CAD build for the part. Positions are in the model's coordinates, mm. A direction names the side the tool comes from. Round coordinates to 2 decimals unless told otherwise and drop trailing zeros. Order: outer loops, then holes, each group sorted by start corner. A loop starts at its lowest first (then second) coordinate and runs counter-clockwise, first axis right, second up. Notation, with made-up numbers: M 76,46.25 L 125,46.25 A22 cw 125,62.25 Z; hole C 87.5,-15 d4. An arc over 180 degrees is marked long. Answer as a JSON object with one key per item and string values.
```python
from build123d import *

# Parameters (mm, degrees)
SKETCH1_W                      = 74.3
SKETCH1_H                      = 60
BOSS_EXTRUDE1_DEPTH            = 1.6
SKETCH2_W                      = 1.9
SKETCH2_H                      = 15
CUT_EXTRUDE1_DEPTH             = 2.6
F_3_2_3_2_DIAMETER_HOLE1_D     = 3.2
F_3_2_3_2_DIAMETER_HOLE1_DEPTH = 60
F_3_2_3_2_DIAMETER_HOLE1_TIP   = 0.96137699
SKETCH6_W                      = 70.5
SKETCH6_H                      = 45
BOSS_EXTRUDE2_DEPTH            = 2
SKETCH7_W                      = 57.288
SKETCH7_H                      = 38.192
BOSS_EXTRUDE3_DEPTH            = 0.5


with BuildPart() as part:
    # Sketch1 → Boss-Extrude1 (new body)
    with BuildSketch(Plane.XY):
        with Locations((37.15, 30)):
            Rectangle(SKETCH1_W, SKETCH1_H)
    extrude(amount=BOSS_EXTRUDE1_DEPTH)

    # Sketch2 → Cut-Extrude1 (cut, through all)
    with BuildSketch(Plane.XY.offset(1.6)):
        with Locations((0.95, 15)):
            Rectangle(SKETCH2_W, SKETCH2_H)
    extrude(amount=-CUT_EXTRUDE1_DEPTH, mode=Mode.SUBTRACT)

    # Ø3.2 (3.2) Diameter Hole1
    with Locations(Plane.XY.offset(1.6)):
        with Locations((4, 56), (70.3, 56), (70.3, 4), (4, 4)):
            Hole(F_3_2_3_2_DIAMETER_HOLE1_D / 2, depth=F_3_2_3_2_DIAMETER_HOLE1_DEPTH)
            with Locations((0, 0, -(F_3_2_3_2_DIAMETER_HOLE1_DEPTH + F_3_2_3_2_DIAMETER_HOLE1_TIP / 2))):  # 118° drill point
                Cone(0, F_3_2_3_2_DIAMETER_HOLE1_D / 2, F_3_2_3_2_DIAMETER_HOLE1_TIP, mode=Mode.SUBTRACT)

    # Sketch6 → Boss-Extrude2 (add)
    with BuildSketch(Plane.XY.offset(1.6)):
        with Locations((37.15, 30)):
            Rectangle(SKETCH6_W, SKETCH6_H)
    extrude(amount=BOSS_EXTRUDE2_DEPTH)

    # Sketch7 → Boss-Extrude3 (add)
    with BuildSketch(Plane.XY.offset(3.6)):
        with Locations((39.936, 30)):
            Rectangle(SKETCH7_W, SKETCH7_H)
    extrude(amount=BOSS_EXTRUDE3_DEPTH)


solid = part.part
```
Item 1: Saw through at A-A on x = 70.3. List the corners of the cut face in (y, z).
Worked answers:
{"outline": "M 0,0 L 2.4,0 L 2.4,1.6 L 0,1.6 Z; M 5.6,0 L 54.4,0 L 54.4,1.6 L 52.5,1.6 L 52.5,3.6 L 7.5,3.6 L 7.5,1.6 L 5.6,1.6 Z; M 57.6,0 L 60,0 L 60,1.6 L 57.6,1.6 Z"}
Item 2: Saw through at D-D on y = 28. List the corners of the cut face in (x, z), and give its area (3 significant figures).
Worked answers:
{"outline": "M 0,0 L 74.3,0 L 74.3,1.6 L 72.4,1.6 L 72.4,3.6 L 68.58,3.6 L 68.58,4.1 L 11.29,4.1 L 11.29,3.6 L 1.9,3.6 L 1.9,1.6 L 0,1.6 Z", "area": "289 mm2"}
Item 3: Wall check: line 1 along Y through (x, z) = (70.3, 0.7); line 2 along Z through (x, y) = (49, 8.5); line 3 along Z through (x, y) = (13, 4). Give the ranges that are in metal, low to high. Write a range as [from, to].
Worked answers:
{"line 1": "y = [0, 2.4], [5.6, 54.4], [57.6, 60]", "line 2": "z = [0, 3.6]", "line 3": "z = [0, 1.6]"}
Item 4: 3-axis set-ups, long thin cutter, end or side, ignore diameter. For faces 4 (the flat face through (1, 7.5, 1)), 5 (the flat face through (37, 52.5, 3)), 6 (the flat face through (37, 7.5, 3)), 7 (the cylindrical face through (71.9, 4.07, 0.79)): which of +Z, -Z, +X, -X, +Y, -Y reach the whole face in a straight line?
Worked answers:
{"face 4": "+Z, -Z, -X", "face 5": "+Z, +X, -X, +Y", "face 6": "+Z, +X, -X, -Y", "face 7": "+Z, -Z"}
Item 5: Saw through at B-B on y = 56. List the corners of the cut face in (x, z).
Worked answers:
{"outline": "M 0,0 L 2.4,0 L 2.4,1.6 L 0,1.6 Z; M 5.6,0 L 68.7,0 L 68.7,1.6 L 5.6,1.6 Z; M 71.9,0 L 74.3,0 L 74.3,1.6 L 71.9,1.6 Z"}
Item 6: Two-plate mould, pull along X, no slides. Class faces 1 (the cylindrical face through (5.27, 3.03, 0.79)), 2 (the flat face through (0, 4, 1)), 3 (the flat face through (72.4, 30, 3)): released by +X, released by -X, zero draft, split by the parting line, or undercut.
Worked answers:
{"face 1": "undercut", "face 2": "released by -X", "face 3": "released by +X"}
Item 7: Drop flat-ended pins along their axis: pin 1 Ø2.5 at (x, y) = (4, 56) entering from -Z; pin 2 Ø1.6 at (x, z) = (23.5, 2.5) entering from +Y; pin 3 Ø1.6 at (x, z) = (29, 2.5) entering from -Y; pin 4 Ø1.6 at (y, z) = (28, 3) entering from +X. Give the stop position or say it passes through.
Worked answers:
{"pin 1": "passes through", "pin 2": "stops at y = 52.5", "pin 3": "stops at y = 7.5", "pin 4": "stops at x = 72.4"}
Item 8: Saw through at C-C on x = 24.5. List the corners of the cut face in (y, z), and give its area (3 significant figures).
Worked answers:
{"outline": "M 0,0 L 60,0 L 60,1.6 L 52.5,1.6 L 52.5,3.6 L 49.1,3.6 L 49.1,4.1 L 10.9,4.1 L 10.9,3.6 L 7.5,3.6 L 7.5,1.6 L 0,1.6 Z", "area": "205 mm2"}
